Autodesk Inventor part; units mm, degrees
ref_plane "YZ Plane" through (0, 0, 0) normal (1, 0, 0) x (0, 1, 0)
ref_plane "XZ Plane" through (0, 0, 0) normal (0, 1, 0) x (-1, 0, 0)
ref_plane "XY Plane" through (0, 0, 0) normal (0, 0, 1) x (1, 0, 0)
sketch "Sketch1" plane through (0, 0, 0) normal (0, 0, 1) x (1, 0, 0)
  line L0 (-137.5, 125) -> (162.5, 125)
  line L1 (162.5, 125) -> (162.5, -125)
  line L2 (162.5, -125) -> (-137.5, -125)
  line L3 (-137.5, -125) -> (-137.5, 125)
  point P0 (0, 0)
  dimension "d0" = 300
  dimension "d1" = 250
  dimension "d2" = 162.5
  dimension "d3" = 125
extrude "Extrusion1" add sketch "Sketch1" along normal blind 10
sketch "Sketch4" plane through (-137.5, 125, 0) normal (0, 1, 0) x (1, 0, 0)
  circle A0 centre (288, -5) radius 3.5
  circle A1 centre (150, -5) radius 3.5
  circle A2 centre (12, -5) radius 3.5
  line L0 (300, 0) -> (300, -10)
  line L1 (0, 0) -> (0, -10)
  line L2 (0, 0) -> (300, 0)
  point P0 (137.5, 0)
  dimension "d6" = 7
  dimension "d7" = 7
  dimension "d8" = 7
  dimension "d9" = 12
  dimension "d10" = 12
  dimension "d12" = 150
  dimension "d13" = 5
  dimension "d14" = 5
  dimension "d15" = 5
extrude "Extrusion2" cut sketch "Sketch4" against normal blind 10
thread "Thread1"
thread "Thread2"
thread "Thread3"
properties part number "Base"
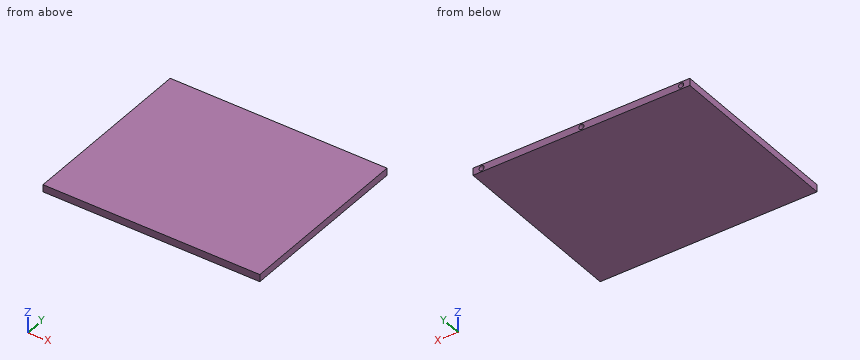
Could you check a few things on this model? Use its own coordinates, in mm. Give positions to 0.01 mm unless a question says otherwise; leave off trailing zeros. Order: outer loops, then holes, each group sorted by start corner. A loop starts at its lowest first (then second) coordinate and runs counter-clockwise, first axis right, second up.
1. I need wall thicknesses on L1, parallel to X at y = 120.5, z = 5; L2, parallel to Z at x = 12.5, y = 120.75; L3, parallel to Y at x = 149, z = 7.25. Which ranges of each line are inside material? Lowest first, please.
2. Will this pin go through, and if not, where does the flat tip stop? P1, Ø3.5, axis at x = 150.5, z = 4.5, coming from the +Y side.
3. Suppose I cut it at A-A (x = -125.5). List the corners of the cut face in (y, z) for me.
Solved:
1. L1: x = -137.5 to -129, -122 to 9, 16 to 147, 154 to 162.5
1. L2: z = 0 to 1.5, 8.5 to 10
1. L3: y = -125 to 115
2. P1: stops at y = 115
3. outline: (-125, 0) - (125, 0) - (125, 1.5) - (115, 1.5) - (115, 8.5) - (125, 8.5) - (125, 10) - (-125, 10) - close
